from build123d import *

# Parameters (mm, degrees)
BOSS_EXTRUDE1_DEPTH                            = 2
BOSS_EXTRUDE3_DEPTH                            = 15
BOSS_EXTRUDE4_DEPTH                            = 15
CSK_FOR_M3_5_FLAT_HEAD_MACHINE_SCREW1_AT_COUNT = 2
CSK_FOR_M3_5_FLAT_HEAD_MACHINE_SCREW1_AT_PITCH = 42.426406871
CSK_FOR_M3_5_FLAT_HEAD_MACHINE_SCREW_2_COUNT   = 2
CSK_FOR_M3_5_FLAT_HEAD_MACHINE_SCREW_2_PITCH   = 60
CSK_FOR_M3_5_FLAT_HEAD_MACHINE_SCREW_3_COUNT   = 2
CSK_FOR_M3_5_FLAT_HEAD_MACHINE_SCREW_3_PITCH   = 42.426406871


with BuildPart() as part:
    # Sketch1 → Boss-Extrude1 (new body)
    with BuildSketch(Plane(origin=(0, 0, 0), x_dir=(1, 0, 0), z_dir=(0, 1, 0))):
        with BuildLine():
            Line((-7.5, 55.75), (-7.5, 27.5))
            ThreePointArc((-7.5, 27.5), (-13.357864376, 13.357864376), (-27.5, 7.5))
            Line((-27.5, 7.5), (-55.75, 7.5))
            Line((-55.75, 7.5), (-55.75, -7.5))
            Line((-55.75, -7.5), (-27.5, -7.5))
            ThreePointArc((-27.5, -7.5), (-13.357864376, -13.357864376), (-7.5, -27.5))
            Line((-7.5, -27.5), (-7.5, -55.75))
            Line((-7.5, -55.75), (7.5, -55.75))
            Line((7.5, -55.75), (7.5, -27.5))
            ThreePointArc((7.5, -27.5), (13.357864376, -13.357864376), (27.5, -7.5))
            Line((27.5, -7.5), (55.75, -7.5))
            Line((55.75, -7.5), (55.75, 7.5))
            Line((55.75, 7.5), (27.5, 7.5))
            ThreePointArc((27.5, 7.5), (13.357864376, 13.357864376), (7.5, 27.5))
            Line((7.5, 27.5), (7.5, 55.75))
            Line((7.5, 55.75), (-7.5, 55.75))
        make_face()
    extrude(amount=BOSS_EXTRUDE1_DEPTH)

    # Sketch3 → Boss-Extrude3 (add)
    with BuildSketch(Plane(origin=(7.5, 0, 0), x_dir=(0, 0, -1), z_dir=(1, 0, 0))):
        Polygon((55.75, 2), (55.75, 8.45), (52.4, 8.45), (51.8, 7.85), (51.8, 6.95), (52.8, 6.95), (52.8, 2), align=None)
    boss_extrude3 = extrude(amount=-BOSS_EXTRUDE3_DEPTH)

    # Mirror1: Boss-Extrude3 across plane
    add(boss_extrude3.mirror(Plane.XY))

    # Sketch6 → Boss-Extrude4 (add)
    with BuildSketch(Plane(origin=(0, 0, -7.5), x_dir=(-1, 0, 0), z_dir=(0, 0, -1))):
        Polygon((55.75, 2), (55.75, 8.45), (52.4, 8.45), (51.8, 7.85), (51.8, 6.95), (52.8, 6.95), (52.8, 2), align=None)
    boss_extrude4 = extrude(amount=-BOSS_EXTRUDE4_DEPTH)

    # Mirror2: Boss-Extrude4 across plane
    add(boss_extrude4.mirror(Plane(origin=(0, 0, 0), x_dir=(0, 0, 1), z_dir=(1, 0, 0))))

    # Sketch9 → CSK for M3.5 Flat Head Machine Screw1 (revolve, cut)
    with BuildSketch(Plane(origin=(0, 2, 30), x_dir=(0, 0, 1), z_dir=(1, 0, 0))):
        Polygon((0, 0), (0, 2), (1.95, 2), (1.95, 2.15), (4.1, 0), align=None)
    csk_for_m3_5_flat_head_machine_screw1 = revolve(axis=Axis((0, 8.35, 30), (0, -1, 0)), mode=Mode.SUBTRACT)

    # CSK for M3.5 Flat Head Machine Screw1 at: CSK for M3.5 Flat Head Machine Screw1 ×2
    with Locations(*[Vector(-0.707106781, 0, -0.707106781) * (i * CSK_FOR_M3_5_FLAT_HEAD_MACHINE_SCREW1_AT_PITCH) for i in range(1, CSK_FOR_M3_5_FLAT_HEAD_MACHINE_SCREW1_AT_COUNT)]):
        add(csk_for_m3_5_flat_head_machine_screw1, mode=Mode.SUBTRACT)

    # CSK for M3.5 Flat Head Machine Screw 2: CSK for M3.5 Flat Head Machine Screw1 ×2
    with Locations(*[(0, 0, -i * CSK_FOR_M3_5_FLAT_HEAD_MACHINE_SCREW_2_PITCH) for i in range(1, CSK_FOR_M3_5_FLAT_HEAD_MACHINE_SCREW_2_COUNT)]):
        add(csk_for_m3_5_flat_head_machine_screw1, mode=Mode.SUBTRACT)

    # CSK for M3.5 Flat Head Machine Screw 3: CSK for M3.5 Flat Head Machine Screw1 ×2
    with Locations(*[Vector(0.707106781, 0, -0.707106781) * (i * CSK_FOR_M3_5_FLAT_HEAD_MACHINE_SCREW_3_PITCH) for i in range(1, CSK_FOR_M3_5_FLAT_HEAD_MACHINE_SCREW_3_COUNT)]):
        add(csk_for_m3_5_flat_head_machine_screw1, mode=Mode.SUBTRACT)


solid = part.part
Here's how the part is built. I have some questions about the finished solid (model axes, mm). A direction names the side the tool comes from. Round coordinates to 2 decimals unless told otherwise and drop trailing zeros. Loops run counter-clockwise (first coordinate to the right, second up) from the corner with the lowest first, then second, coordinate; pieces in that order, holes last.
1. If we section it at C-C on x = 0: Write out the boundary of the cut face in (y, z), plus the area to 3 significant figures.
Answer list:
outline: (0, -55.75) - (8.45, -55.75) - (8.45, -52.4) - (7.85, -51.8) - (6.95, -51.8) - (6.95, -52.8) - (2, -52.8) - (2, -34.1) - (0, -32.1) - close; (0, -27.9) - (2, -25.9) - (2, 25.9) - (0, 27.9) - close; (0, 32.1) - (2, 34.1) - (2, 52.8) - (6.95, 52.8) - (6.95, 51.8) - (7.85, 51.8) - (8.45, 52.4) - (8.45, 55.75) - (0, 55.75) - close
area: 239 mm2
2. If we section it at A-A on y = 4.25: Write out the boundary of the cut face in (x, z).
Answer list:
outline: (-55.75, -7.5) - (-52.8, -7.5) - (-52.8, 7.5) - (-55.75, 7.5) - close; (-7.5, -55.75) - (7.5, -55.75) - (7.5, -52.8) - (-7.5, -52.8) - close; (-7.5, 52.8) - (7.5, 52.8) - (7.5, 55.75) - (-7.5, 55.75) - close; (52.8, -7.5) - (55.75, -7.5) - (55.75, 7.5) - (52.8, 7.5) - close
3. If I drill on line 1 along Z through (x, y) = (4.5, 7); line 2 along Z through (x, y) = (-5.5, 5.25); line 3 along Y through (x, z) = (20, -0.5), over which ranges is the centre line in solid material (lowest first)?
Answer list:
line 1: z = -55.75 to -51.8, 51.8 to 55.75
line 2: z = -55.75 to -52.8, 52.8 to 55.75
line 3: y = 0 to 2
4. For P1, Ø6, axis at x = -14.5, z = -7.5, coming from the +Y side; P2, Ø2.5, axis at x = -45, y = 3, coming from the -Z side; P3, Ø5, axis at y = 1, z = 13, coming from the +X side, each with a flat end and sliding along its axis, tell me the tip position at first contact or that it passes through.
Answer list:
P1: stops at y = 2
P2: stops at z = -7.5
P3: stops at x = 16.96
5. If we section it at B-B on z = -30: Write out the boundary of the cut face in (x, y), plus the area to 3 significant figures.
Answer list:
outline: (-7.5, 0) - (-2.1, 0) - (-4.1, 2) - (-7.5, 2) - close; (2.1, 0) - (7.5, 0) - (7.5, 2) - (4.1, 2) - close
area: 17.6 mm2
6. If we section it at D-D on z = 0: Write out the boundary of the cut face in (x, y), plus the area to 3 significant figures.
Answer list:
outline: (-55.75, 0) - (-32.1, 0) - (-34.1, 2) - (-52.8, 2) - (-52.8, 6.95) - (-51.8, 6.95) - (-51.8, 7.85) - (-52.4, 8.45) - (-55.75, 8.45) - close; (-27.9, 0) - (27.9, 0) - (25.9, 2) - (-25.9, 2) - close; (32.1, 0) - (55.75, 0) - (55.75, 8.45) - (52.4, 8.45) - (51.8, 7.85) - (51.8, 6.95) - (52.8, 6.95) - (52.8, 2) - (34.1, 2) - close
area: 239 mm2
7. Which directions (+Z, -Z, +X, -X, +Y, -Y) give clear straight access to the entire face, cutting with the end or side of a thin tool? Please do faces 1 (the face through (45.7, 1.7, 7.5)), 2 (the face through (0, 4, -55.75)), 3 (the face through (0, 5, -52.8)), 4 (the face through (7.5, 1.7, -45.7)).
Answer list:
face 1: +Z, +X, +Y, -Y
face 2: -Z, +X, -X, +Y, -Y
face 3: +X, -X
face 4: -Z, +X, +Y, -Y
8. We'd pull the mould along X, two halves only. Please class faces 5 (the face through (-52.8, 5, 0)), 6 (the face through (-54, 8.45, 0)), 7 (the face through (13.514, 0.986, -13.203)), 8 (the face through (-55.75, 4, 0)): +X half, -X half, draft (parallel to the pull), parting line (faces both ways), or undercut.
Answer list:
face 5: undercut
face 6: draft
face 7: +X half
face 8: -X half
